Can you work these out from the drawing? Everything is in mm from the part's minimum corner. Round coordinates to 2 decimals unless told otherwise and drop trailing zeros. Order: outer loops, then holes, each group sorted by start corner. A loop starts at its lowest first (then second) coordinate and runs counter-clockwise, first axis right, second up. Notation, with made-up numbers: (10, 67.25) - (50, 67.25) arc R23 cw to (50, 89.25) - close; hole circle Ø4 at (-12.5, -1). An arc over 180 degrees is marked (long way). Answer as a JSON object with one key per item and string values.
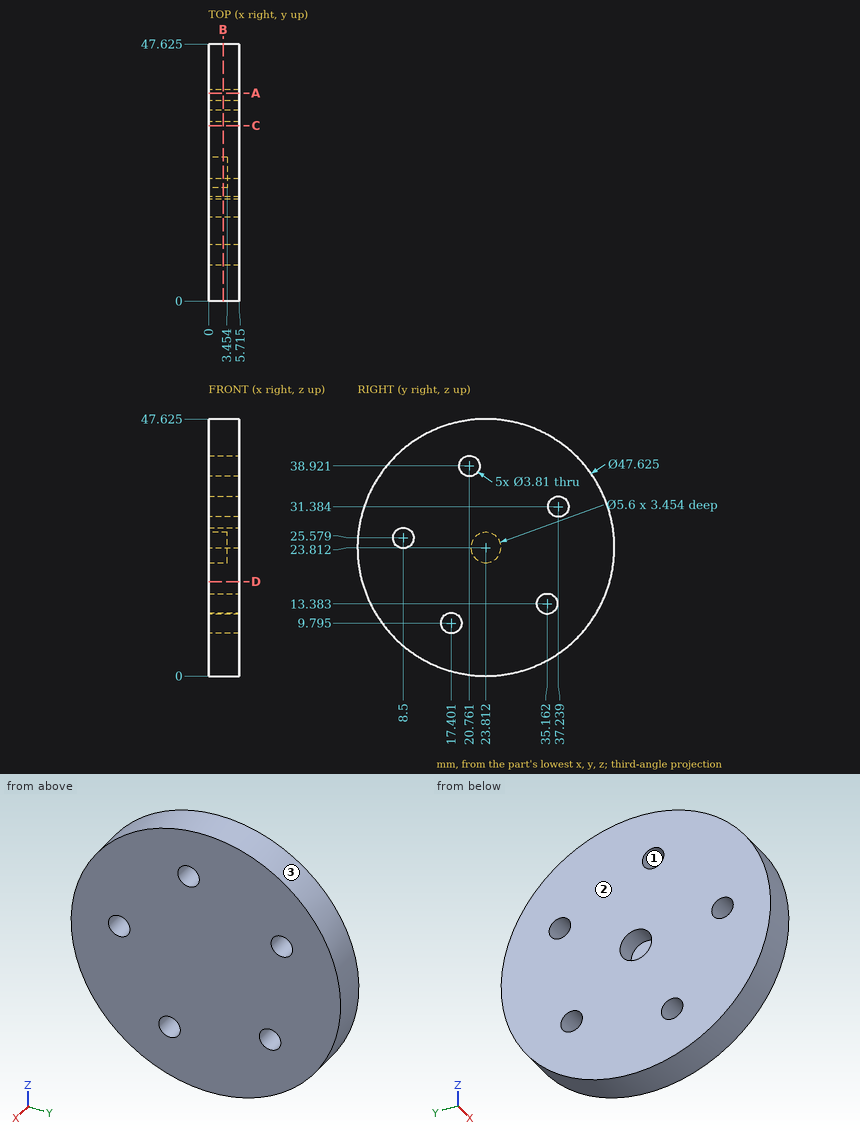
1. Imagine slicing it at A-A (y = 38.5). List the corners of the cut face in (x, z) for me (1 decimal).
Responses:
{"outline": "(0, 5.1) - (5.7, 5.1) - (5.7, 30) - (0, 30) - close; (0, 32.8) - (5.7, 32.8) - (5.7, 42.6) - (0, 42.6) - close"}
2. Imagine slicing it at D-D (z = 17.5). List the corners of the cut face in (x, y) for me (1 decimal).
Responses:
{"outline": "(0, 0.9) - (5.7, 0.9) - (5.7, 46.8) - (0, 46.8) - close"}
3. If I drill on L1, parallel to Y at x = 4, z = 25.5 (1 decimal); L2, parallel to Z at x = 2.05, y = 38.5 (1 decimal); L3, parallel to Y at x = 3.35, z = 39.5 (1 decimal), over which ranges is the centre line in solid material (lowest first)? Write a range as [from, to].
Responses:
{"L1": "[0.1, 6.6], [10.4, 47.6]", "L2": "[5.1, 30], [32.8, 42.6]", "L3": "[5.9, 18.9], [22.6, 41.7]"}
4. Imagine slicing it at C-C (y = 32.5). List the corners of the cut face in (x, z) for me (1 decimal).
Responses:
{"outline": "(0, 1.6) - (5.7, 1.6) - (5.7, 46) - (0, 46) - close"}
5. For P1, Ø3, axis at x = 4, z = 22, coming from the -Y side; P2, Ø4.5, axis at y = 8.5, z = 25.58, coming from the +X side (1 decimal); P3, Ø1.5, axis at x = 1.5, z = 43, coming from the +Y side; P4, Ø3, axis at x = 1.5, z = 24, coming from the +Y side (1 decimal), each with a flat end and sliding along its axis, tell me the tip position at first contact or that it passes through.
Responses:
{"P1": "y = 0", "P2": "x = 5.7", "P3": "y = 38.88", "P4": "y = 47.6"}
6. Imagine slicing it at B-B (x = 2.7). List the corners of the cut face in (y, z) for me (1 decimal).
Responses:
{"outline": "circle Ø47.6 at (23.8, 23.8); hole circle Ø3.8 at (8.5, 25.6); hole circle Ø3.8 at (17.4, 9.8); hole circle Ø3.8 at (20.8, 38.9); hole circle Ø5.6 at (23.8, 23.8); hole circle Ø3.8 at (35.2, 13.4); hole circle Ø3.8 at (37.2, 31.4)"}
7. Thinking about a two-plate mould opening in Y: for the marked faces 1, 2 and 3, which applies, pulls with the +Y half, pulls with the -Y half, needs draft (parallel to the pull), parting line crosses it, or undercut?
Responses:
{"face 1": "undercut", "face 2": "needs draft", "face 3": "parting line crosses it"}
